Autodesk Inventor part; units mm, degrees
ref_plane "YZ Plane" through (0, 0, 0) normal (1, 0, 0) x (0, 1, 0)
ref_plane "XZ Plane" through (0, 0, 0) normal (0, 1, 0) x (-1, 0, 0)
ref_plane "XY Plane" through (0, 0, 0) normal (0, 0, 1) x (1, 0, 0)
sketch "Sketch1" plane through (0, 0, 0) normal (0, 0, 1) x (1, 0, 0)
  circle A0 centre (0, 0) radius 17.8
  dimension "d0" = 35.6
extrude "Extrusion1" add sketch "Sketch1" along normal blind 2.54
sketch "Sketch2" plane through (0, 0, 2.54) normal (0, 0, 1) x (1, 0, 0)
  circle A0 centre (0, 0) radius 17.8
  line L0 (-24.92, 0) -> (24.92, 0)
  line L1 (0, -24.92) -> (0, 24.92)
  circle A1 centre (0, 14.84) radius 1
  circle A2 centre (-10.4935, 10.4935) radius 1
  circle A3 centre (-14.84, 0) radius 1
  circle A4 centre (-10.4935, -10.4935) radius 1
  circle A5 centre (0, -14.84) radius 1
  circle A6 centre (10.4935, -10.4935) radius 1
  circle A7 centre (14.84, 0) radius 1
  circle A8 centre (10.4935, 10.4935) radius 1
  circle A9 centre (0, 0) radius 3
  dimension "d3" = 2
  dimension "d4" = 14.84
  dimension "d7" = 360
  dimension "d9" = 6
extrude "Extrusion2" cut sketch "Sketch2" against normal blind 2.54 contours A7 L0 | L0 A7 | A1 L1 | L1 A1 | A5 L1 | L1 A5 | A3 L0 | L0 A3 | A9 L1 L0 | L0 L1 A9 | L1 L0 A9 | A9 L0 L1 | A2 | A4 | A6 | A8
properties part number "ServoFutabaS3003_circularArm"
Can you work these out from the model? Positions are in its coordinate system, mm. Give positions to 0.01 mm unless a question says otherwise; leave off trailing zeros. Loops run counter-clockwise (first coordinate to the right, second up) from the corner with the lowest first, then second, coordinate; pieces in that order, holes last. Notation, with made-up numbers: (48.5, 39) -> (65.5, 39) arc R30 cw to (65.5, 64) -> close; hole circle Ø1 at (48.25, -28). An arc over 180 degrees is marked (long way). Write item = value, one per line.
1) Suppose I cut it at D-D on x = 14.5. Write out the boundary of the cut face in (y, z).
Check result:
outline = (-10.32, 0) -> (-0.94, 0) -> (-0.94, 2.54) -> (-10.32, 2.54) -> close; (0.94, 0) -> (10.32, 0) -> (10.32, 2.54) -> (0.94, 2.54) -> close
2) Suppose I cut it at A-A on x = 0. Write out the boundary of the cut face in (y, z).
Check result:
outline = (-17.8, 0) -> (-15.84, 0) -> (-15.84, 2.54) -> (-17.8, 2.54) -> close; (-13.84, 0) -> (-3, 0) -> (-3, 2.54) -> (-13.84, 2.54) -> close; (3, 0) -> (13.84, 0) -> (13.84, 2.54) -> (3, 2.54) -> close; (15.84, 0) -> (17.8, 0) -> (17.8, 2.54) -> (15.84, 2.54) -> close
3) Will these pins go through, and if not, where does the flat tip stop? pin 1 (2.5 mm diameter, centred on x = -14.84, y = 0, fed in from +Z); pin 2 (1.5 mm diameter, centred on x = -13.5, z = 1, fed in from +Y); pin 3 (1.2 mm diameter, centred on x = -10.49, y = 10.49, fed in from +Z).
Check result:
pin_1 = 2.54
pin_2 = 12.42
pin_3 = through
4) Thinking about a two-plate mould opening in Y: for faces 1 (the flat face through (4, 0, 2.54)), 2 (the cylindrical face through (-3.859, 17.377, 1.252)), 3 (the cylindrical face through (-0.13, -13.85, 1.29)), which applies, released by +Y, released by -Y, zero draft, split by the parting line, or undercut?
Check result:
face_1 = zero draft
face_2 = split by the parting line
face_3 = undercut
5) I need wall thicknesses on L1, parallel to Y at x = 0, z = 0.65; L2, parallel to X at y = -10, z = 1.75; L3, parallel to Y at x = -0.5, z = 0.5. Which ranges of each line are inside material? Lowest first, please. Write a range as from..to.
Check result:
L1 = -17.8..-15.84, -13.84..-3, 3..13.84, 15.84..17.8
L2 = -14.73..-11.36, -9.62..9.62, 11.36..14.73
L3 = -17.79..-15.71, -13.97..-2.96, 2.96..13.97, 15.71..17.79
6) Suppose I cut it at C-C on z = 2. Give the number of separate pieces and of enclosed holes in the cut face, then the cut area to 3 significant figures.
Check result:
separate_pieces = 1
enclosed_holes = 9
area = 942 mm2
